```python
from build123d import *

# Parameters (mm, degrees)
F0_W     = 894.08
F0_H     = 640.08
F0_R     = 61.341
F1_DEPTH = 25.4


with BuildPart() as f1:
    # F0 (on Front) → F1 (new body)
    with BuildSketch(Plane.XZ):
        Rectangle(F0_W, F0_H)
        with Locations((-338.185633, -210.813498)):
            Circle(F0_R, mode=Mode.SUBTRACT)
        with Locations((338.000492, -211.000518)):
            Circle(F0_R, mode=Mode.SUBTRACT)
        with BuildLine():
            ThreePointArc((-27.94, 127), (-9.979488, 119.560512), (-2.54, 101.6))
            Line((-2.54, 101.6), (-2.54, -101.6))
            ThreePointArc((-2.54, -101.6), (-9.979488, -119.560512), (-27.94, -127))
            Line((-27.94, -127), (-231.14, -127))
            ThreePointArc((-231.14, -127), (-249.100512, -119.560512), (-256.54, -101.6))
            Line((-256.54, -101.6), (-256.54, 101.6))
            ThreePointArc((-256.54, 101.6), (-249.100512, 119.560512), (-231.14, 127))
            Line((-231.14, 127), (-27.94, 127))
        make_face(mode=Mode.SUBTRACT)
        with Locations((-338.000518, 211.000492)):
            Circle(F0_R, mode=Mode.SUBTRACT)
        with Locations((338.000492, 211.000492)):
            Circle(F0_R, mode=Mode.SUBTRACT)
    extrude(amount=F1_DEPTH)


solid = f1.part
```
Read the model definition and answer for the solid it produces. Units are mm, in the model's axes. A direction names the side the tool comes from. Give positions to 0.01 mm unless a question says otherwise; leave off trailing zeros. Order: outer loops, then holes, each group sorted by start corner. A loop starts at its lowest first (then second) coordinate and runs counter-clockwise, first axis right, second up. Notation, with made-up numbers: (-1.5, -19.5) -> (46.5, -19.5) arc R28 ccw to (46.5, 18.5) -> close; hole circle Ø2 at (-6, 50). An arc over 180 degrees is marked (long way). One line per item, written item: value. Start each with the question number.
(1) The part is cut by section C-C (y = -18.5). Determine the outline of the cut face in (x, z), and give its area (3 significant figures).
(2) The part is cut by section B-B (x = -381.5). Determine the outline of the cut face in (y, z).
(3) The part is cut by section A-A (z = 27). Determine the outline of the cut face in (x, y), and give its area (3 significant figures).
(4) A tool of negligible diameter and unlimited length cuts with its end or side. For faces 4 (the flat face through (93, 0, 4)), 5 (the flat face through (-256.54, -13, -1)), from which of +Z, -Z, +X, -X, +Y, -Y can it reach the whole face along a straight path? Write none if from no direction.
(5) The part is cut by section D-D (x = -17.5). Determine the outline of the cut face in (y, z), and give its area (3 significant figures).
(6) For a pull along Z with two mould halves and no side action, classify faces 1 (the flat face through (-6, -13, -320.04)), 2 (the flat face through (447.04, -13, -4)), 3 (the cylindrical face through (-9.78, -12.52, -119.36)) as released by +Z, released by -Z, zero draft, split by the parting line, or undercut.
(7) Straight lines are drawn through the part: L1, parallel to X at y = -13.5, z = 210; L2, parallel to X at y = -3.75, z = 61; L3, parallel to Z at x = -370.5, y = -23.5. For each, find the intervals that lie inside material, in ascending order.
Taken from the geometry:
1. outline: (-447.04, -320.04) -> (447.04, -320.04) -> (447.04, 320.04) -> (-447.04, 320.04) -> close; hole circle Ø122.68 at (-338.19, -210.81); hole circle Ø122.68 at (-338, 211); hole (-256.54, -101.6) arc R25.4 ccw to (-231.14, -127) -> (-27.94, -127) arc R25.4 ccw to (-2.54, -101.6) -> (-2.54, 101.6) arc R25.4 ccw to (-27.94, 127) -> (-231.14, 127) arc R25.4 ccw to (-256.54, 101.6) -> close; hole circle Ø122.68 at (338, -211); hole circle Ø122.68 at (338, 211)
1. area: 461,000 mm^2
2. outline: (-25.4, -320.04) -> (0, -320.04) -> (0, -254.25) -> (-25.4, -254.25) -> close; (-25.4, -167.38) -> (0, -167.38) -> (0, 167.75) -> (-25.4, 167.75) -> close; (-25.4, 254.25) -> (0, 254.25) -> (0, 320.04) -> (-25.4, 320.04) -> close
3. outline: (-447.04, -25.4) -> (-256.54, -25.4) -> (-256.54, 0) -> (-447.04, 0) -> close; (-2.54, -25.4) -> (447.04, -25.4) -> (447.04, 0) -> (-2.54, 0) -> close
3. area: 16,300 mm^2
4. face 4: +Z, -Z, +X, -X, +Y
4. face 5: +Y, -Y
5. outline: (-25.4, -320.04) -> (0, -320.04) -> (0, -124.76) -> (-25.4, -124.76) -> close; (-25.4, 124.76) -> (0, 124.76) -> (0, 320.04) -> (-25.4, 320.04) -> close
5. area: 9,920 mm^2
6. face 1: released by -Z
6. face 2: zero draft
6. face 3: undercut
7. L1: -447.04 to -399.33, -276.67 to 276.67, 399.33 to 447.04
7. L2: -447.04 to -256.54, -2.54 to 447.04
7. L3: -320.04 to -262.95, -158.67 to 158.98, 263.02 to 320.04
